```python
from build123d import *

# Parameters (mm, degrees)
SKETCH1_R                     = 76.73
BOSS_EXTRUDE1_DEPTH           = 10
BOSS_EXTRUDE1_OTHER_WAY_DEPTH = 8
BOSS_EXTRUDE1_OTHER_WAY_TAPER = 70
SKETCH2_R                     = 17.9565
CUT_EXTRUDE1_DEPTH            = 18
SKETCH3_R                     = 74.247849381
CUT_EXTRUDE2_DEPTH            = 10
BOSS_EXTRUDE2_START           = 5
SKETCH4_R                     = 19.169573719
SKETCH4_R_2                   = 17.9565
BOSS_EXTRUDE2_DEPTH           = 5


with BuildPart() as part:
    # Sketch1 → Boss-Extrude1 (new body)
    with BuildSketch(Plane.XY):
        Circle(SKETCH1_R)
    extrude(amount=BOSS_EXTRUDE1_DEPTH)

    # Sketch1 → Boss-Extrude1 other way (add)
    with BuildSketch(Plane.XY):
        Circle(SKETCH1_R)
    extrude(amount=-BOSS_EXTRUDE1_OTHER_WAY_DEPTH, taper=BOSS_EXTRUDE1_OTHER_WAY_TAPER)

    # Sketch2 → Cut-Extrude1 (cut)
    with BuildSketch(Plane(origin=(0, 0, -8), x_dir=(-1, 0, 0), z_dir=(0, 0, -1))):
        Circle(SKETCH2_R)
    extrude(amount=-CUT_EXTRUDE1_DEPTH, mode=Mode.SUBTRACT)

    # Sketch3 → Cut-Extrude2 (cut)
    with BuildSketch(Plane.XY.offset(10)):
        Circle(SKETCH3_R)
    extrude(amount=-CUT_EXTRUDE2_DEPTH, mode=Mode.SUBTRACT)

    # Sketch4 → Boss-Extrude2 (add)
    with BuildSketch(Plane(origin=(0, 0, -8), x_dir=(-1, 0, 0), z_dir=(0, 0, -1)).offset(BOSS_EXTRUDE2_START)):
        with Locations(Location((0, 0, 0), (0, 0, 180))):
            Circle(SKETCH4_R)
        Circle(SKETCH4_R_2, mode=Mode.SUBTRACT)
    extrude(amount=-BOSS_EXTRUDE2_DEPTH)


solid = part.part
```
Here's how the part is built. I have some questions about the finished solid (model axes, mm). A direction names the side the tool comes from. Coordinates: 2 decimals unless noted, no trailing zeros. Order: outer loops, then holes, each group sorted by start corner. A loop starts at its lowest first (then second) coordinate and runs counter-clockwise, first axis right, second up.
Item 1: Which directions (+Z, -Z, +X, -X, +Y, -Y) give clear straight access to the entire face, cutting with the end or side of a thin tool? Please do faces 4 (the face through (-16.634, -74.905, 4.93)), 5 (the face through (24, 1, -8)), 6 (the face through (70.82, 22.3, 5.07)).
Response values:
face 4: +Z, -Z
face 5: -Z
face 6: +Z
Item 2: If we section it at A-A, the plane x = 0: List the corners of the cut face in (y, z) for me.
Response values:
outline: (-76.73, 0) - (-54.75, -8) - (-19.17, -8) - (-19.17, -13) - (-17.96, -13) - (-17.96, 0) - (-74.25, 0) - (-74.25, 10) - (-76.73, 10) - close; (17.96, -13) - (19.17, -13) - (19.17, -8) - (54.75, -8) - (76.73, 0) - (76.73, 10) - (74.25, 10) - (74.25, 0) - (17.96, 0) - close
Item 3: Thinking about a two-plate mould opening in Y: for faces 1 (the face through (15, -15, 0)), 2 (the face through (18.284, -5.758, -10.535)), 3 (the face through (-40, 63, 10)), which applies, pulls with the +Y half, pulls with the -Y half, needs draft (parallel to the pull), parting line crosses it, or undercut?
Response values:
face 1: undercut
face 2: parting line crosses it
face 3: needs draft
Item 4: If we section it at C-C, the plane z = -11: List the corners of the cut face in (x, y) for me.
Response values:
outline: circle Ø38.34 at (0, 0); hole circle Ø35.91 at (0, 0)
Item 5: I need wall thicknesses on probe 1 along Y at (x, z) = (0, -9.25); probe 2 along X at (y, z) = (-48, 5); probe 3 along Y at (x, z) = (0, 2.5). Which ranges of each line are inside material? Lowest first, please.
Response values:
probe 1: y = -19.17 to -17.96, 17.96 to 19.17
probe 2: x = -59.86 to -56.65, 56.65 to 59.86
probe 3: y = -76.73 to -74.25, 74.25 to 76.73
Item 6: I'm going to push flat-ended pins straight in: pin 1 Ø6 at (y, z) = (58, 6.5) entering from +X; pin 2 Ø12 at (x, y) = (-36, 0.5) entering from -Z; pin 3 Ø4 at (x, y) = (36.5, 15) entering from +Z. Where does each tip first touch, or does it pass through?
Response values:
pin 1: stops at x = 53.5
pin 2: stops at z = -8
pin 3: stops at z = 0
Item 7: If we section it at B-B, the plane z = 7.25: List the corners of the cut face in (x, y) for me.
Response values:
outline: circle Ø153.46 at (0, 0); hole circle Ø148.5 at (0, 0)
